Geometry check sheet. Reference: the model listing, model coordinates, mm. A direction names the side the tool comes from. Round coordinates to 2 decimals unless told otherwise and drop trailing zeros. Order: outer loops, then holes, each group sorted by start corner. A loop starts at its lowest first (then second) coordinate and runs counter-clockwise, first axis right, second up. Notation, with made-up numbers: (-28, 67.5) - (6, 67.5) arc R30 cw to (6, 103.5) - close; hole circle Ø5 at (4, -33). An arc over 180 degrees is marked (long way). Use a Markdown table: item, result. Add a question column.
(1) Section check B-B on x = -15.5. Record the boundary of the cut face in (y, z).
(2) Access from +Z, -Z, +X, -X, +Y, -Y to the whole of each face (thin tool, end or side, straight path). Record for faces 1 (the face through (-1, 5, 0)), 2 (the face through (-34, 10, -19)).
(3) Gauge pin test, flat ends, axial feed: P1, Ø2.5, axis at x = 33.5, z = 20.7, coming from the -Y side; P2, Ø2, axis at x = 9.5, y = 5.5, coming from the +Z side; P3, Ø5, axis at x = 19, z = 10, coming from the -Y side; P4, Ø4, axis at x = 33.5, z = -20.7, coming from the -Y side. Record the tip position at first contact, or that the pin passes through.
(4) Section check A-A on z = 20.7. Give the number of separate pieces and of enclosed holes in the cut face, then the cut area to 3 significant figures.
(5) Section check D-D on z = 12. Record the boundary of the cut face in (x, y).
(6) Mould release check, pull along X, two halves, no side actions. Record for faces 3 (the face through (-32.8, 10, 22.2)), 4 (the face through (32.3, 5.4, 21.6)), 5 (the face through (-34.61, 5.44, -21.71)): released by +X, released by -X, zero draft, split by the parting line, or undercut.
(7) Thickness scan on line 1 along Z through (x, y) = (-33.5, 6.25); line 2 along Z through (x, y) = (33.5, 3.75); line 3 along X through (y, z) = (7, 20.7). Record the ranges inside material, lowest first. Write a range as [from, to].
```python
from build123d import *

# Parameters (mm, degrees)
SKETCH3_W           = 80
SKETCH3_H           = 60
BOSS_EXTRUDE1_DEPTH = 5
SKETCH5_R           = 3.5
BOSS_EXTRUDE2_DEPTH = 5
SKETCH6_R           = 1.5
SKETCH6_R_2         = 3.2
CUT_EXTRUDE1_DEPTH  = 11
CHAMFER1_SIZE       = 1


with BuildPart() as part:
    # Sketch3 → Boss-Extrude1 (new body)
    with BuildSketch(Plane(origin=(0, 0, 0), x_dir=(1, 0, 0), z_dir=(0, 1, 0))):
        Rectangle(SKETCH3_W, SKETCH3_H)
    extrude(amount=BOSS_EXTRUDE1_DEPTH)

    # Sketch5 → Boss-Extrude2 (add)
    with BuildSketch(Plane(origin=(0, 5, 0), x_dir=(1, 0, 0), z_dir=(0, 1, 0))):
        with Locations((33.5, 20.7)):
            Circle(SKETCH5_R)
        with Locations((33.5, -20.7)):
            Circle(SKETCH5_R)
        with Locations((-33.5, -20.7)):
            Circle(SKETCH5_R)
        with Locations((-33.5, 20.7)):
            Circle(SKETCH5_R)
    extrude(amount=BOSS_EXTRUDE2_DEPTH)

    # Sketch6 → Cut-Extrude1 (cut, through all)
    with BuildSketch(Plane(origin=(0, 0, 0), x_dir=(1, 0, 0), z_dir=(0, 1, 0))):
        with Locations((33.5, -20.7)):
            Circle(SKETCH6_R)
        with Locations((33.5, 20.7)):
            Circle(SKETCH6_R)
        with Locations((-33.5, -20.7)):
            Circle(SKETCH6_R)
        with Locations((-33.5, 20.7)):
            Circle(SKETCH6_R)
        with Locations((4.995, 7.825)):
            Circle(SKETCH6_R_2)
    extrude(amount=CUT_EXTRUDE1_DEPTH, mode=Mode.SUBTRACT)

    # Chamfer1
    chamfer1_edges = [part.edges().sort_by_distance(p)[0] for p in [
        (-40, 5, 0),
        (30, 5, -20.7),
        (0, 5, 30),
        (30, 5, 20.7),
        (-37, 5, 20.7),
        (-37, 5, -20.7),
        (32, 0, -20.7),
        (-35, 0, 20.7),
        (-35, 0, -20.7),
        (1.795, 0, -7.825),
        (1.795, 5, -7.825),
        (32, 0, 20.7),
        (40, 5, 0),
        (0, 0, 30),
        (-40, 0, 0),
        (0, 0, -30),
        (40, 0, 0),
        (40, 2.5, 30),
        (-40, 2.5, 30),
        (-40, 2.5, -30),
        (40, 2.5, -30),
        (0, 5, -30),
    ]]
    chamfer(chamfer1_edges, length=CHAMFER1_SIZE)


solid = part.part
```
Check sheet entries:
| question | item | result |
|---|---|---|
| 1 | outline | (0, -29) - (1, -30) - (4, -30) - (5, -29) - (5, 29) - (4, 30) - (1, 30) - (0, 29) - close |
| 2 | face 1 | +Y |
| 2 | face 2 | +Z, -Z, +X, -X, +Y |
| 3 | P1 | passes through |
| 3 | P2 | stops at z = 29.5 |
| 3 | P3 | stops at y = 0 |
| 3 | P4 | stops at y = 0.5 |
| 4 | separate pieces | 3 |
| 4 | enclosed holes | 0 |
| 4 | area | 408 mm2 |
| 5 | outline | (-40, 1) - (-39, 0) - (39, 0) - (40, 1) - (40, 4) - (39, 5) - (-39, 5) - (-40, 4) - close |
| 6 | face 3 | zero draft |
| 6 | face 4 | undercut |
| 6 | face 5 | undercut |
| 7 | line 1 | z = [-24.2, -22.2], [-19.2, -17.2], [17.2, 19.2], [22.2, 24.2] |
| 7 | line 2 | z = [-30, -22.2], [-19.2, 19.2], [22.2, 30] |
| 7 | line 3 | x = [-37, -35], [-32, -30], [30, 32], [35, 37] |
